The drawing under review shows one solid part. Ordinate dimensions are in mm from its lowest x, y, z. Round coordinates to 2 decimals unless told otherwise and drop trailing zeros. Order: outer loops, then holes, each group sorted by start corner. A loop starts at its lowest first (then second) coordinate and runs counter-clockwise, first axis right, second up. Notation, with made-up numbers: (61, 63) - (78, 63) arc R28 cw to (78, 89) - close; hole circle Ø2 at (-13.5, 80.5). An arc over 180 degrees is marked (long way). One line per question, with ' | ' between items.
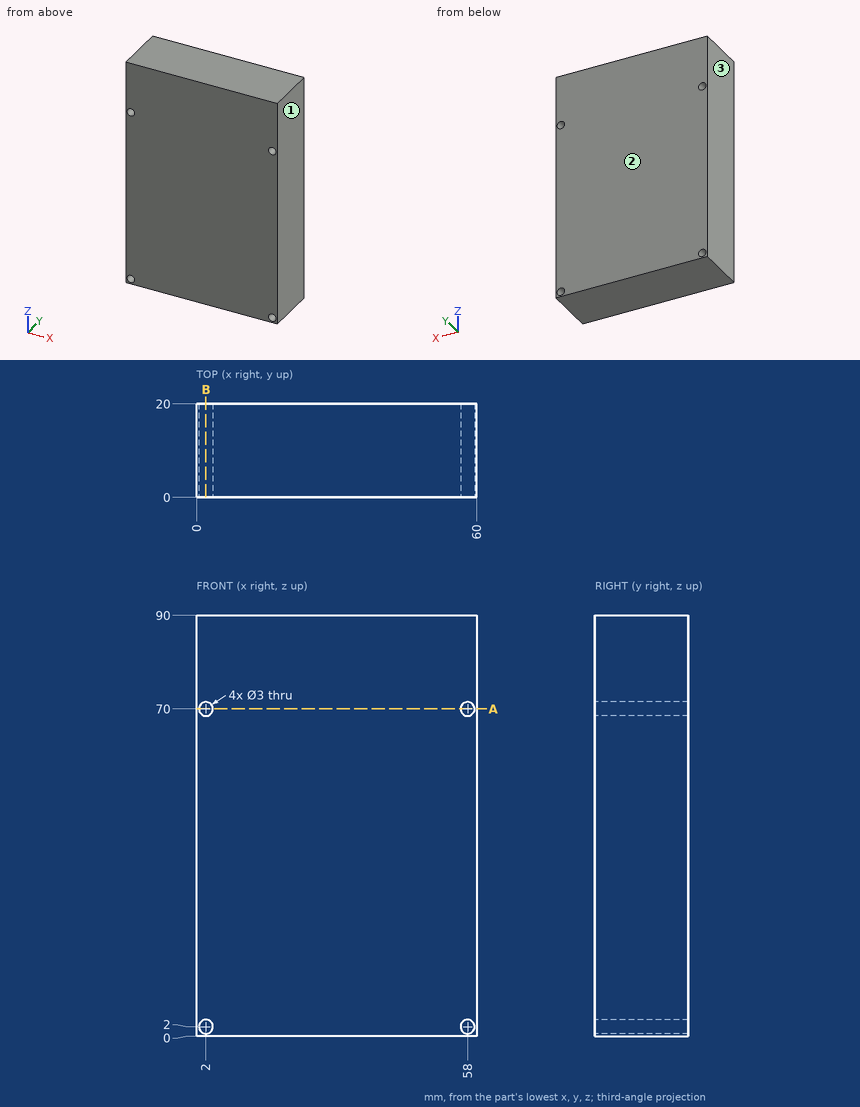
(1) For probe 1 along X at (y, z) = (10.75, 2); probe 2 along Z at (x, y) = (2, 5), list the stretches that pass through material, from the lowest coordinate up. Write a range as [from, to].
Output values:
probe 1: [0, 0.5], [3.5, 56.5], [59.5, 60] | probe 2: [0, 0.5], [3.5, 68.5], [71.5, 90]
(2) Mouldability with a two-part tool opening along X and no side actions: class the marked faces 1, 2 and 3 as released by +X, released by -X, zero draft, split by the parting line, or undercut.
Output values:
face 1: released by +X | face 2: zero draft | face 3: released by -X
(3) We need section A-A on z = 70. State the section outline as (x, y) points.
Output values:
outline: (0, 0) - (0.5, 0) - (0.5, 20) - (0, 20) - close; (3.5, 0) - (56.5, 0) - (56.5, 20) - (3.5, 20) - close; (59.5, 0) - (60, 0) - (60, 20) - (59.5, 20) - close
(4) We need section B-B on x = 2. State the section outline as (y, z) points, plus the area to 3 significant figures.
Output values:
outline: (0, 0) - (20, 0) - (20, 0.5) - (0, 0.5) - close; (0, 3.5) - (20, 3.5) - (20, 68.5) - (0, 68.5) - close; (0, 71.5) - (20, 71.5) - (20, 90) - (0, 90) - close | area: 1,680 mm^2
